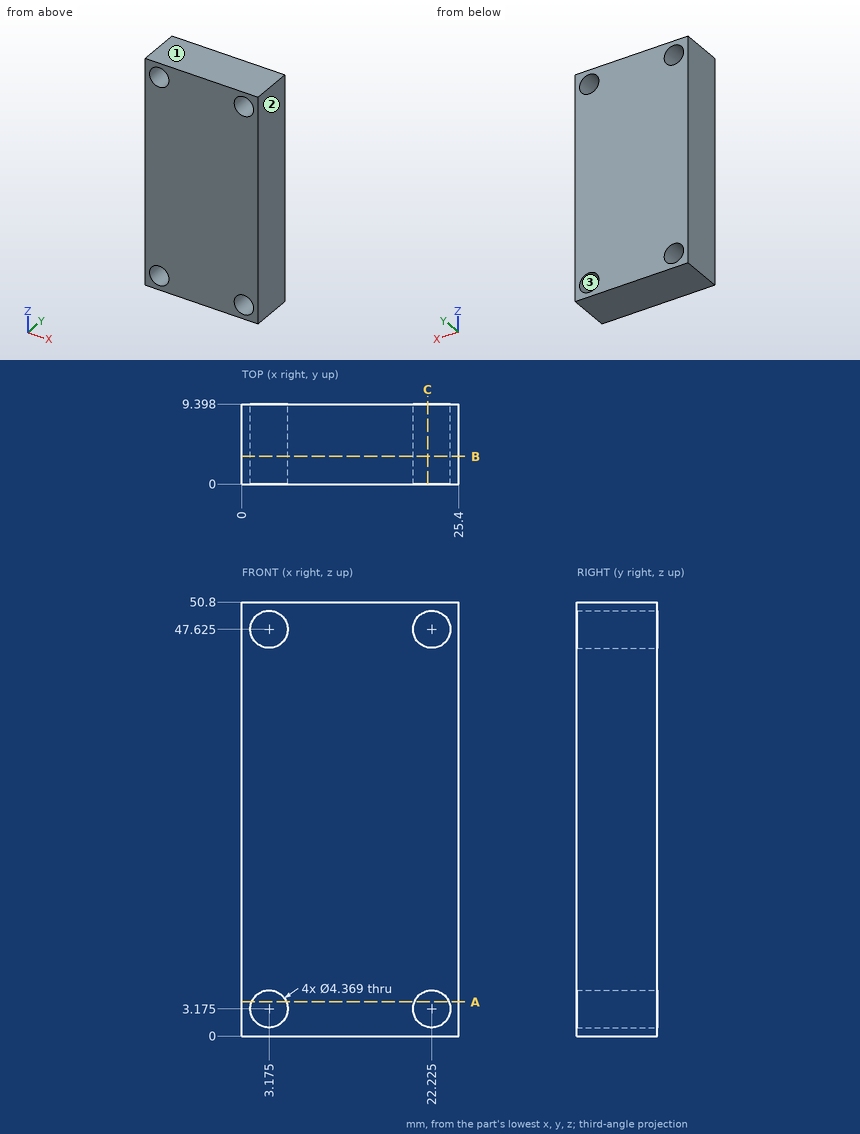
Design review of the part shown in the three views and the two pictorial views. Dimensions are in mm from the part's minimum x, y and z. Give positions to 0.01 mm unless a question says otherwise; leave off trailing zeros. Order: outer loops, then holes, each group sorted by start corner. A loop starts at its lowest first (then second) coordinate and runs counter-clockwise, first axis right, second up. Notation, with made-up numbers: M 33,82 L 77,82 A33 ccw 77,115 Z; hole C 11.5,-12 d3. An arc over 180 degrees is marked long. Answer in a Markdown table with one row per item. Add a question column.
(1) Wall thickness on probe 1 along Z at (x, y) = (22, 2); probe 2 along X at (y, z) = (3, 3); probe 3 along X at (y, z) = (0.5, 46) (1 decimal): over which ranges is each line inside the solid? List them lowest first. Write a range as [from, to].
(2) Consider section A-A on z = 4. State the section outline as (x, y) points, and give its area (3 significant figures).
(3) Mouldability with a two-part tool opening along X and no side actions: class the marked faces 1, 2 and 3 as +X half, -X half, draft (parallel to the pull), parting line (faces both ways), or undercut.
(4) Consider section C-C on x = 21.75. State the section outline as (y, z) points.
(5) Consider section B-B on y = 3.25. State the section outline as (x, z) points (1 decimal).
Evaluation:
| question | item | result |
|---|---|---|
| 1 | probe 1 | z = [0, 1], [5.35, 45.45], [49.8, 50.8] |
| 1 | probe 2 | x = [0, 1], [5.35, 20.05], [24.4, 25.4] |
| 1 | probe 3 | x = [0, 1.7], [4.6, 20.8], [23.7, 25.4] |
| 2 | outline | M 0,0 L 1.15,0 L 1.15,9.4 L 0,9.4 Z; M 5.2,0 L 20.2,0 L 20.2,9.4 L 5.2,9.4 Z; M 24.25,0 L 25.4,0 L 25.4,9.4 L 24.25,9.4 Z |
| 2 | area | 163 mm^2 |
| 3 | face 1 | draft |
| 3 | face 2 | +X half |
| 3 | face 3 | undercut |
| 4 | outline | M 0,0 L 9.4,0 L 9.4,1.04 L 0,1.04 Z; M 0,5.31 L 9.4,5.31 L 9.4,45.49 L 0,45.49 Z; M 0,49.76 L 9.4,49.76 L 9.4,50.8 L 0,50.8 Z |
| 5 | outline | M 0,0 L 25.4,0 L 25.4,50.8 L 0,50.8 Z; hole C 3.2,3.2 d4.4; hole C 3.2,47.6 d4.4; hole C 22.2,3.2 d4.4; hole C 22.2,47.6 d4.4 |
